CAD build for the part. Positions are in the model's coordinates, mm. A direction names the side the tool comes from. Coordinates: 2 decimals unless noted, no trailing zeros. Loops run counter-clockwise (first coordinate to the right, second up) from the corner with the lowest first, then second, coordinate; pieces in that order, holes last. Notation, with made-up numbers: (62, -3.75) - (68, -3.75) arc R12 ccw to (68, 5.25) - close; hole circle Ø10 at (-12.75, 7.5). An arc over 180 degrees is marked (long way). Put each result on its own line as item: value.
```python
from build123d import *

# Parameters (mm, degrees)
F0_R     = 50.8
F1_DEPTH = 12.7
F2_R     = 33.491229
F3_DEPTH = 38.1
F4_R     = 29.55091
F5_DEPTH = 25.4
F6_R     = 5.08


with BuildPart() as f1:
    # F0 (on Front) → F1 (new body)
    with BuildSketch(Plane.XZ):
        Circle(F0_R)
    extrude(amount=F1_DEPTH)

    # F2 (on Front) → F3 (join)
    with BuildSketch(Plane.XZ):
        Circle(F2_R)
    extrude(amount=-F3_DEPTH)

    # F4 (on face) → F5 (join)
    with BuildSketch(Plane(origin=(0, 38.1, 0), x_dir=(-1, 0, 0), z_dir=(0, 1, 0))):
        Circle(F4_R)
    extrude(amount=F5_DEPTH)

    # F6
    f6_edges = [f1.edges().sort_by_distance(p)[0] for p in [
        (29.55091, 63.5, 0),
    ]]
    fillet(f6_edges, radius=F6_R)


solid = f1.part
```
Q1. Slice it at B-B, the plane z = 0. Give the cut face in (x, y), then the cut area to 3 significant figures.
Determined:
outline: (-50.8, -12.7) - (50.8, -12.7) - (50.8, 0) - (33.49, 0) - (33.49, 38.1) - (29.55, 38.1) - (29.55, 58.42) arc R5.08 ccw to (24.47, 63.5) - (-24.47, 63.5) arc R5.08 ccw to (-29.55, 58.42) - (-29.55, 38.1) - (-33.49, 38.1) - (-33.49, 0) - (-50.8, 0) - close
area: 5,330 mm2
Q2. Tool access for faces 1 (the cylindrical face through (-11.012, -6.261, -49.592)), 2 (the flat face through (0, 38.1, -30)): list every direction of +Z, -Z, +X, -X, +Y, -Y with a clear straight run to the whole face (end or side of a thin tool).
Determined:
face 1: +Y, -Y
face 2: +Y
Q3. Slice it at D-D, the plane z = -32. Give the cut face in (x, y), then the cut area to 3 significant figures.
Determined:
outline: (-39.45, -12.7) - (39.45, -12.7) - (39.45, 0) - (9.88, 0) - (9.88, 38.1) - (-9.88, 38.1) - (-9.88, 0) - (-39.45, 0) - close
area: 1,760 mm2
Q4. Slice it at C-C, the plane y = 34. Give the cut face in (x, z).
Determined:
outline: circle Ø66.98 at (0, 0)
Q5. Slice it at A-A, the plane x = 0. Give the cut face in (y, z).
Determined:
outline: (-12.7, -50.8) - (0, -50.8) - (0, -33.49) - (38.1, -33.49) - (38.1, -29.55) - (58.42, -29.55) arc R5.08 ccw to (63.5, -24.47) - (63.5, 24.47) arc R5.08 ccw to (58.42, 29.55) - (38.1, 29.55) - (38.1, 33.49) - (0, 33.49) - (0, 50.8) - (-12.7, 50.8) - close
Q6. Wall check: L1, parallel to Y at x = -27, z = 20.5; L2, parallel to X at y = -1, z = -0.5; L3, parallel to Y at x = 30, z = 2. Give the ranges that are in metal, low to high. Write a range as from..to.
Determined:
L1: -12.7..0
L2: -50.8..50.8
L3: -12.7..38.1
Q7. Pin check, flat tips, straight feed: pin 1 Ø5 at (x, z) = (-33, -10) entering from +Y; pin 2 Ø6 at (y, z) = (33.5, 14) entering from -X; pin 3 Ø5 at (y, z) = (14, -11) entering from +X. Stop position of each tip, or through.
Determined:
pin 1: y = 38.1
pin 2: x = -31.63
pin 3: x = 32.39
